Geometry check sheet. Reference: drawing and pictorial views, mm from the part's lowest x, y, z. A direction names the side the tool comes from. Coordinates: 2 decimals unless noted, no trailing zeros. Write each loop counter-clockwise with the first axis right and the second up, starting at its lowest first coordinate (ties: lowest second). Pieces come first, ordered by that corner, then holes. Notation, with made-up numbers: M 47.25,-27 L 60.25,-27 A13 ccw 60.25,-19 Z; hole C -4.75,-9.5 d11. An arc over 180 degrees is marked long. One line per item, written item: value.
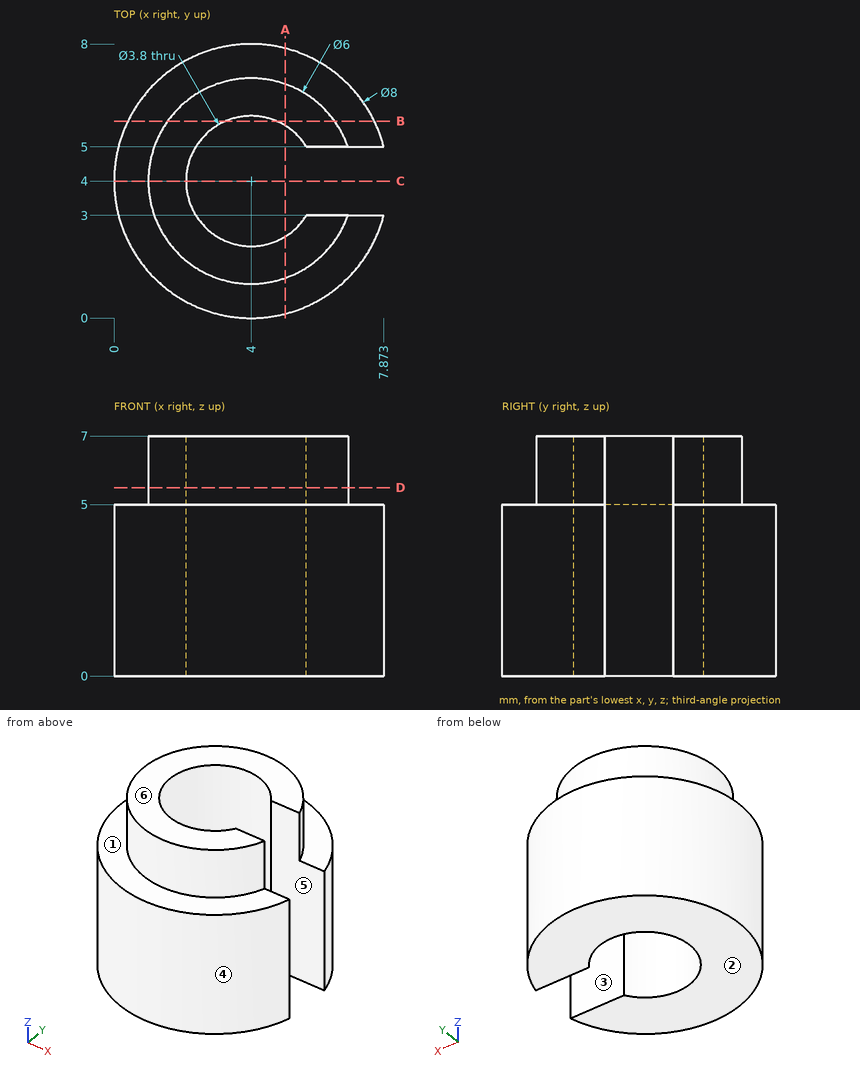
Item 1: Cross-section at C-C, the plane y = 4. Enter the section's corners in (x, z), and give its area (3 significant figures).
The answers:
outline: M 0,0 L 2.1,0 L 2.1,7 L 1,7 L 1,5 L 0,5 Z
area: 12.7 mm²
Item 2: Access from +Z, -Z, +X, -X, +Y, -Y to the whole of each face (thin tool, end or side, straight path). Record for the marked faces 1, 2 and 3.
The answers:
face 1: +Z
face 2: -Z, +X, -X, +Y, -Y
face 3: +Z, -Z, +X
Item 3: Cross-section at B-B, the plane y = 5.75. Enter the section's corners in (x, z), and give its area (3 significant figures).
The answers:
outline: M 0.4,0 L 3.26,0 L 3.26,7 L 1.56,7 L 1.56,5 L 0.4,5 Z; M 4.74,0 L 7.6,0 L 7.6,5 L 6.44,5 L 6.44,7 L 4.74,7 Z
area: 35.4 mm²
Item 4: Draft check along Y on the marked faces 4, 5 and 6. Enter one of: released by +Y, released by -Y, zero draft, split by the parting line, or undercut.
The answers:
face 4: split by the parting line
face 5: undercut
face 6: zero draft
Item 5: Go/stop test with flat-tipped pins: P1, Ø4, axis at y = 6.5, z = 5.5, coming from the -X side; P2, Ø3, axis at x = 1, z = 4, coming from the +Y side; P3, Ø1.8, axis at x = 6, z = 3.5, coming from the +Y side. Record where each tip stops, or that it passes through.
The answers:
P1: stops at x = 0.04
P2: stops at y = 7.71
P3: stops at y = 7.85
Item 6: Scan lines: line 1 (Y direction, x = 4, z = 4.75); line 2 (X direction, y = 4, z = 1.5); line 3 (Z direction, x = 2, y = 7.25). Record each from-to range of solid material in increasing order.
The answers:
line 1: y = 0 to 2.1, 5.9 to 8
line 2: x = 0 to 2.1
line 3: z = 0 to 5
Item 7: Cross-section at A-A, the plane x = 5. Enter the section's corners in (y, z), and give its area (3 significant figures).
The answers:
outline: M 0.13,0 L 2.38,0 L 2.38,7 L 1.17,7 L 1.17,5 L 0.13,5 Z; M 5.62,0 L 7.87,0 L 7.87,5 L 6.83,5 L 6.83,7 L 5.62,7 Z
area: 27.4 mm²
Item 8: Cross-section at D-D, the plane z = 5.5. Enter the section's corners in (x, y), and give its area (3 significant figures).
The answers:
outline: M 5.62,3 A1.9 cw long 5.62,5 L 6.83,5 A3 ccw long 6.83,3 Z
area: 14.7 mm²
